```python
from build123d import *

# Parameters (mm, degrees)
REVOLVE_ONTO_SKETCH002_ROLL_ANGLE = 90
REVOLVE_ROLL_ANGLE                = -90
SKETCH001_R                       = 0.275
SWEEP_ROLL_ANGLE                  = -90


with BuildPart() as revolve_body:
    # Sketch002 as drawn → Revolve (revolve)
    with BuildSketch(Plane.XY):
        with BuildLine():
            Line((-2.5, 1.2), (-2, 1.2))
            ThreePointArc((-1.6, 1.12065), (-1.796103, 1.179971), (-2, 1.2))
            Line((-1.6, 1.12065), (-1.5, 1.07935))
            ThreePointArc((-1.5, 1.07935), (-1.303897, 1.020029), (-1.1, 1))
            Line((1.1, 1), (-1.1, 1))
            ThreePointArc((1.1, 1), (1.303897, 1.020029), (1.5, 1.07935))
            Line((1.6, 1.12065), (1.5, 1.07935))
            ThreePointArc((2, 1.2), (1.796103, 1.179971), (1.6, 1.12065))
            Line((2.5, 1.2), (2, 1.2))
            ThreePointArc((3, 0.7), (2.853553, 1.053553), (2.5, 1.2))
            ThreePointArc((3, 0.7), (3.050926, 0.335979), (3.2, 0))
            Line((3.2, 0), (-3.2, 0))
            ThreePointArc((-3.2, 0), (-3.045646, 0.326695), (-2.999778, 0.685095))
            ThreePointArc((-2.5, 1.2), (-2.858785, 1.048244), (-2.999778, 0.685095))
        make_face()
    revolve(axis=Axis((0, 0, 0), (1, 0, 0)))


with BuildPart() as revolve_body_1:
    # Revolve onto Sketch002 roll: moved
    add(revolve_body.part.rotate(Axis((0, 0, 0), (1, 0, 0)), REVOLVE_ONTO_SKETCH002_ROLL_ANGLE))


with BuildPart() as revolve_body_2:
    # Revolve onto Sketch002 placement: moved
    add(revolve_body_1.part)


with BuildPart() as revolve_body_3:
    # Revolve roll: moved
    add(revolve_body_2.part.rotate(Axis((0, 0, 0), (1, 0, 0)), REVOLVE_ROLL_ANGLE))


with BuildPart() as revolve_body_4:
    # Revolve placement: moved
    add(revolve_body_3.part.moved(Location((0, 0, 1.3))))


with BuildPart() as resistor:
    # Sweep: sweep along a path in Sketch
    with BuildLine(Plane.XY) as sweep_path:
        Line((-3.9, 3.6), (-3.9, 0.6))
        ThreePointArc((-3.9, 0.6), (-3.724264, 0.175736), (-3.3, 0))
        Line((-3.3, 0), (3.3, 0))
        ThreePointArc((3.3, 0), (3.724264, 0.175736), (3.9, 0.6))
        Line((3.9, 0.6), (3.9, 3.6))
    # Sketch001 → Sweep (sweep)
    with BuildSketch(Plane.YZ):
        Circle(SKETCH001_R)
    sweep(path=sweep_path.line)


with BuildPart() as resistor_1:
    # Sweep roll: moved
    add(resistor.part.rotate(Axis((0, 0, 0), (1, 0, 0)), SWEEP_ROLL_ANGLE))


with BuildPart() as resistor_2:
    # Sweep placement: moved
    add(resistor_1.part.moved(Location((0, 0, 1.3))))

    # Fusion: union Revolve body
    add(revolve_body_4.part)


solid = resistor_2.part
```
Model file for the job. Use its own axes, mm. Round coordinates to 2 decimals unless told otherwise and drop trailing zeros. Order: outer loops, then holes, each group sorted by start corner. A loop starts at its lowest first (then second) coordinate and runs counter-clockwise, first axis right, second up. Notation, with made-up numbers: (-13.75, -1) -> (31.25, -1) arc R14 ccw to (31.25, 21) -> close; hole circle Ø6 at (66.5, 1). An arc over 180 degrees is marked (long way). Use one line per item in the form item = value.
Item 1: Drill centre lines: line 1 (X direction, y = -0.2, z = -0.3); line 2 (Y direction, x = 1.5, z = 1.25); line 3 (Z direction, x = 3.5, y = 0.15). Where is each one in solid material? Low to high.
Returned:
line_1 = -4.09 to -3.71, 3.71 to 4.09
line_2 = -1.08 to 1.08
line_3 = 1.01 to 1.51
Item 2: Cut at A-A, the plane z = -1.7. Write the cut outline in (x, y) (3 decimals), and give its area (3 significant figures).
Returned:
outline = circle Ø0.55 at (-3.9, 0); circle Ø0.55 at (3.9, 0)
area = 0.475 mm^2
Item 3: Cut at B-B, the plane x = -1. Write the cut outline in (y, z), and give its area (3 significant figures).
Returned:
outline = circle Ø2 at (0, 1.3)
area = 3.14 mm^2
Item 4: Cut at C-C, the plane z = 0.4. Give the number of separate pieces and of enclosed holes in the cut face, and give its area (3 significant figures).
Returned:
separate_pieces = 3
enclosed_holes = 0
area = 7.41 mm^2
